Can you work these out from the model? Positions are in its coordinate system, mm. Give positions to 0.01 mm unless a question says otherwise; leave off trailing zeros. Loops run counter-clockwise (first coordinate to the right, second up) from the corner with the lowest first, then second, coordinate; pieces in that order, holes last. Notation, with made-up numbers: (-30.75, 49.5) - (-7.75, 49.5) arc R17 cw to (-7.75, 55.5) - close; hole circle Ø11 at (21, -35). An arc over 180 degrees is marked (long way). Answer as a JSON object with one key per item and string values. Group by question number.
Item 1: Suppose I cut it at C-C on z = -8.25. Write out the boundary of the cut face in (x, y).
Item 2: Suppose I cut it at A-A on y = -1.65. Count the separate pieces of the cut face and the enclosed holes in it, and give its area (3 significant figures).
Item 3: Please list where these lines run through material, in increasing order: L1, parallel to Z at x = 5, y = -1.1; L2, parallel to Z at x = 4.5, y = -0.4; L3, parallel to X at y = -0.7, z = -3.5.
Item 4: Thinking about a two-plate mould opening in Z: for faces 1 (the cylindrical face through (1, -1, -2)), 2 (the cylindrical face through (5, -1, -4)), 3 (the flat face through (37, -2, -5)), which applies, pulls with the +Z half, pulls with the -Z half, needs draft (parallel to the pull), parting line crosses it, or undercut?
Item 5: Suppose I cut it at B-B on z = -1. Write out the boundary of the cut face in (x, y).
from build123d import *

# Parameters (mm, degrees)
F0_W     = 75.7
F0_H     = 10
F0_R     = 1
F1_DEPTH = 2
F2_R     = 5
F3_R     = 4.99999
F4_R     = 5
F5_R     = 4.99999


# Not quite as in the source:
# - a fillet or chamfer is up to 0.001 mm smaller than in the source, because OpenCascade refuses the exact size


with BuildPart() as f1:
    # F0 (on Front) → F1 (new body)
    with BuildSketch(Plane.XZ):
        with Locations((37.85, -5)):
            Rectangle(F0_W, F0_H)
        with Locations((5, -5)):
            Circle(F0_R, mode=Mode.SUBTRACT)
        with Locations((70.7, -5)):
            Circle(F0_R, mode=Mode.SUBTRACT)
    extrude(amount=F1_DEPTH)

    # F2
    f2_edges = [f1.edges().sort_by_distance(p)[0] for p in [
        (0, -1, 0),
    ]]
    fillet(f2_edges, radius=F2_R)

    # F3 (radius 5 in the source; OpenCascade refuses exactly that, so slightly less here)
    f3_edges = [f1.edges().sort_by_distance(p)[0] for p in [
        (0, -1, -10),
    ]]
    fillet(f3_edges, radius=F3_R)

    # F4
    f4_edges = [f1.edges().sort_by_distance(p)[0] for p in [
        (75.7, -1, -10),
    ]]
    fillet(f4_edges, radius=F4_R)

    # F5 (radius 5 in the source; OpenCascade refuses exactly that, so slightly less here)
    f5_edges = [f1.edges().sort_by_distance(p)[0] for p in [
        (75.7, -1, 0),
    ]]
    fillet(f5_edges, radius=F5_R)


solid = f1.part
Worked out:
{
 "1": {"outline": "(1.2, -2) - (74.5, -2) - (74.5, 0) - (1.2, 0) - close"},
 "2": {"separate pieces": "1", "enclosed holes": "2", "area": "729 mm2"},
 "3": {"L1": "z = -10 to -6, -4 to 0", "L2": "z = -9.97 to -5.87, -4.13 to -0.03", "L3": "x = 0.23 to 75.47"},
 "4": {"face 1": "pulls with the +Z half", "face 2": "undercut", "face 3": "needs draft"},
 "5": {"outline": "(2, -2) - (73.7, -2) - (73.7, 0) - (2, 0) - close"}
}
